Part model, mm, in its own coordinate system. Face numbers are marked on the shaded views. A direction names the side the tool comes from. Round coordinates to 2 decimals unless told otherwise and drop trailing zeros. Loops run counter-clockwise (first coordinate to the right, second up) from the corner with the lowest first, then second, coordinate; pieces in that order, holes last. Notation, with made-up numbers: (38, 60) -> (51, 60) arc R19 ccw to (51, 88) -> close; hole circle Ø9 at (3, 74). An arc over 180 degrees is marked (long way). Use a Markdown table: item, result. Add a question column.
Item 1: Cut at B-B, the plane z = 15.5. List the corners of the cut face in (x, y), plus the area to 3 significant figures.
Item 2: Flat gauge pins, fed straight in: pin 1 (4 mm diameter, centred on y = -519.5, z = -3.5, fed in from -X); pin 2 (1 mm diameter, centred on x = -55.5, z = 9, fed in from -Y); pin 3 (12 mm diameter, centred on y = -510, z = -17.5, fed in from -X). Where does each tip first touch, or does it go through?
Item 3: Probe line 1 (Z direction, x = -111.5, y = -514.5) (3 decimals); line 2 (X direction, y = -485, z = -15.5); line 3 (Y direction, x = -106, z = 7). List the from-to ranges inside material, lowest first. Write a range as [from, to].
Item 4: Which spindle directions (+Z, -Z, +X, -X, +Y, -Y) get a long thin tool onto all of the face, cutting with end or side? Do the marked faces 1 and 2. Say none if no direction does.
Item 5: Cut at D-D, the plane y = -507.5. List the corners of the cut face in (x, z) (3 decimals), plus the area to 3 significant figures.
Item 6: Cut at C-C, the plane x = -66.5. List the corners of the cut face in (y, z) (3 decimals), plus the area to 3 significant figures.
Item 7: Two-plate mould, pull along Z, no slides. Class the marked faces 3, 4, 5 and 6: pulls with the +Z half, pulls with the -Z half, needs draft (parallel to the pull), parting line crosses it, or undercut.
Item 8: Cut at A-A, the plane y = -531.5. List the corners of the cut face in (x, z) (3 decimals).
Autodesk Inventor part; units mm, degrees
ref_plane "Work Plane1" through (-188.0551, -545.2781, -26.8885) normal (-0.4043748, 0.9145934, 0) x (0, 0, 1)
ref_plane "YZ Plane" through (0, 0, 0) normal (1, 0, 0) x (0, 1, 0)
ref_plane "XZ Plane" through (0, 0, 0) normal (0, 1, 0) x (-1, 0, 0)
sketch "Sketch1" plane through (0, 0, 0) normal (0, 0, 1) x (1, 0, 0)
  line L0 (-7.3059, -465.3624) -> (-4.6413, -482.4725)
  line L1 (-9.4718, -491.3147) -> (-125.6251, -542.6703)
  line L2 (-125.6251, -542.6703) -> (-148.9715, -527.9978)
  line L3 (-148.9715, -527.9978) -> (-7.3059, -465.3624) construction
  line L4 (-7.3059, -465.3624) -> (-10.4732, -462.5969)
  line L5 (-10.4732, -462.5969) -> (-149.0606, -523.8714)
  line L6 (-149.0606, -523.8714) -> (-148.9715, -527.9978)
  line L7 (-9.4718, -491.3147) -> (-4.6413, -482.4725)
  point P0 (0, 0)
  point P1 (-3.6641, -488.7469)
  dimension "d3" = 3.81
  dimension "d6" = 133.35
  dimension "d8" = 6.35
  dimension "d9" = 6.35
extrude "Extrusion1" add sketch "Sketch1" along normal mid plane 44.45
sketch "Sketch2" plane through (-138.2759, -548.2636, 22.225) normal (-0.4043748, 0.9145934, 0) x (0.9145934, 0.4043748, 0)
  line L0 (-1.5872, 10) -> (153.3074, 10) construction
  line L1 (153.3074, 34.45) -> (-1.5872, 34.45) construction
  line L2 (163.3576, 10) -> (-32.3991, 10)
  line L3 (-32.3991, 10) -> (-32.3991, 34.45)
  line L4 (-32.3991, 34.45) -> (163.3576, 34.45)
  line L5 (163.3576, 34.45) -> (163.3576, 10)
  line L6 (163.3576, 6.0918) -> (163.3576, 38.3582) construction
  line L7 (-32.3991, 3.3518) -> (-32.3991, 41.0982) construction
  point P0 (348.1702, 22.225)
ref_plane "Work Plane1" through (-188.0551, -545.2781, -26.8885) normal (-0.4043748, 0.9145934, 0) x (0, 0, 1)
extrude "Extrusion2" cut sketch "Sketch2" along normal up to surface (22.86 mm away)
sketch "Sketch4" plane through (0, 0, 0) normal (0, 0, 1) x (1, 0, 0)
  point P0 (0, 0)
properties part number "BottomGrip"
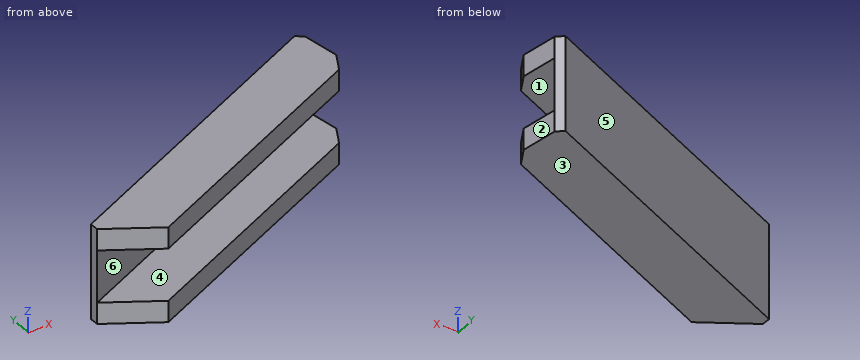
A:
| question | item | result |
|---|---|---|
| 1 | outline | (-149.06, -523.87) -> (-148.97, -528) -> (-125.63, -542.67) -> (-9.47, -491.31) -> (-4.64, -482.47) -> (-7.31, -465.36) -> (-10.47, -462.6) -> close |
| 1 | area | 3,860 mm^2 |
| 2 | pin 1 | stops at x = -143.7 |
| 2 | pin 2 | stops at y = -486.89 |
| 2 | pin 3 | stops at x = -131.26 |
| 3 | line 1 | z = [-22.225, -12.225], [12.225, 22.225] |
| 3 | line 2 | x = [-61.14, -6.02] |
| 3 | line 3 | y = [-509, -504.83] |
| 4 | face 1 | +X, -Y |
| 4 | face 2 | +Z, -Z, +X, +Y |
| 5 | outline | (-112.033, -22.225) -> (-46.079, -22.225) -> (-46.079, -12.225) -> (-102.616, -12.225) -> (-102.616, 12.225) -> (-46.079, 12.225) -> (-46.079, 22.225) -> (-112.033, 22.225) -> close |
| 5 | area | 1,550 mm^2 |
| 6 | outline | (-516.529, -22.225) -> (-487.368, -22.225) -> (-487.368, 22.225) -> (-516.529, 22.225) -> (-516.529, 12.225) -> (-491.532, 12.225) -> (-491.532, -12.225) -> (-516.529, -12.225) -> close |
| 6 | area | 685 mm^2 |
| 7 | face 3 | pulls with the -Z half |
| 7 | face 4 | undercut |
| 7 | face 5 | needs draft |
| 7 | face 6 | undercut |
| 8 | outline | (-143.399, -22.225) -> (-100.361, -22.225) -> (-100.361, -12.225) -> (-143.399, -12.225) -> close; (-143.399, 12.225) -> (-100.361, 12.225) -> (-100.361, 22.225) -> (-143.399, 22.225) -> close |
